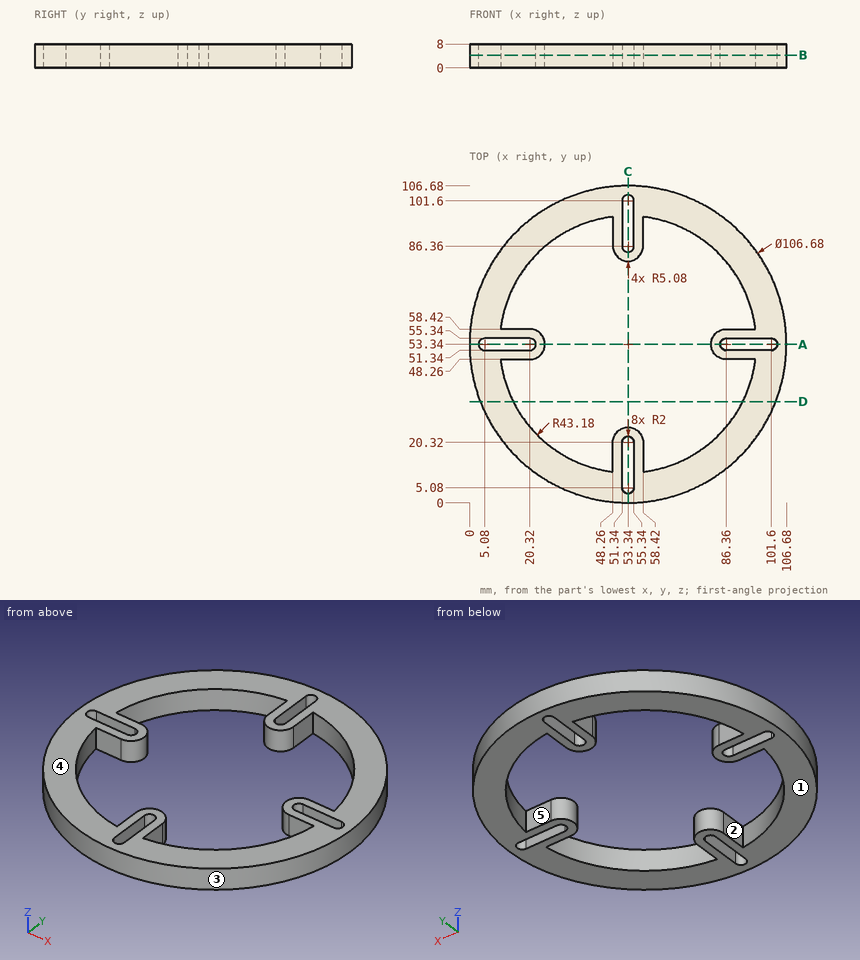
Geometry check sheet. Reference: drawing and pictorial views, mm from the part's lowest x, y, z. A direction names the side the tool comes from. Round coordinates to 2 decimals unless told otherwise and drop trailing zeros. Write each loop counter-clockwise with the first axis right and the second up, starting at its lowest first coordinate (ties: lowest second). Pieces come first, ordered by that corner, then holes.
(1) Section check A-A (y = 53.34). Enter the section's corners in (x, z), plus the area to 3 significant figures.
Returned:
outline: (0, 0) - (3.08, 0) - (3.08, 8) - (0, 8) - close; (22.32, 0) - (25.4, 0) - (25.4, 8) - (22.32, 8) - close; (81.28, 0) - (84.36, 0) - (84.36, 8) - (81.28, 8) - close; (103.6, 0) - (106.68, 0) - (106.68, 8) - (103.6, 8) - close
area: 98.6 mm2
(2) Access from +Z, -Z, +X, -X, +Y, -Y to the whole of each face (thin tool, end or side, straight path). Record for the marked faces 4 and 5.
Returned:
face 4: +Z, +X, -X, +Y, -Y
face 5: +Z, -Z
(3) Material ranges on line 1 (X direction, y = 53, z = 7.75); line 2 (Y direction, x = 53.5, z = 2); line 3 (Y direction, x = 16.5, z = 4.75), recorded low to high.
Returned:
line 1: x = 0 to 3.11, 22.29 to 25.39, 81.29 to 84.39, 103.57 to 106.68
line 2: y = 0 to 3.09, 22.31 to 25.4, 81.28 to 84.37, 103.59 to 106.68
line 3: y = 14.77 to 30.82, 48.26 to 51.34, 55.34 to 58.42, 75.86 to 91.91
(4) Mould release check, pull along Y, two halves, no side actions. Record for the marked faces 1, 2 and 3: pulls with the +Y half, pulls with the -Y half, needs draft (parallel to the pull), parting line crosses it, or undercut.
Returned:
face 1: needs draft
face 2: undercut
face 3: parting line crosses it
(5) Section check B-B (z = 4.25). Give the number of separate pieces and of enclosed holes in the cut face, plus the area to 3 significant figures.
Returned:
separate pieces: 1
enclosed holes: 5
area: 3,360 mm2
(6) Section check D-D (y = 34). Enter the section's corners in (x, z).
Returned:
outline: (3.63, 0) - (14.73, 0) - (14.73, 8) - (3.63, 8) - close; (91.95, 0) - (103.05, 0) - (103.05, 8) - (91.95, 8) - close
(7) Depth check by flat-ended pin: pin 1 Ø4 at (x, z) = (94, 4.5) entering from -Y; pin 2 Ø2 at (x, z) = (93.5, 4.5) entering from +Y; pin 3 Ø1.5 at (x, z) = (83, 4) entering from +Y. Enter the tip coordinate at first touch or a pass-through.
Returned:
pin 1: stops at y = 16.59
pin 2: stops at y = 89.56
pin 3: stops at y = 98.17
